from build123d import *

# Parameters (mm, degrees)
BASE_SHAPE_DEPTH                               = 3
EDGE_RADIUSES_R                                = 3.4
CAMERA_MOUNT_HOLES_REACH                       = 5
SKETCH3_R                                      = 1
CSK_FOR_M2_FLAT_HEAD_MACHINE_SCREW1_AT_2_COUNT = 2
CSK_FOR_M2_FLAT_HEAD_MACHINE_SCREW1_AT_2_PITCH = 22
MILLING_RADIUSES_R                             = 1
SKETCH8_R                                      = 0.5
MILLING_CUTS_1MM_DEPTH                         = 3


with BuildPart() as part:
    # Sketch1 → Base shape (new body)
    with BuildSketch(Plane.XY):
        Polygon((15.5, 6), (-15.5, 6), (-15.5, -6), (-14, -6), (-14, -6.9), (-11.05, -6.9), (-11.05, -5.1), (-12.3, -5.1), (-12.3, -2.9), (-7.7, -2.9), (-7.7, -5.1), (-8.95, -5.1), (-8.95, -6.9), (-6, -6.9), (-6, -6), (6, -6), (6, -6.9), (8.95, -6.9), (8.95, -5.1), (7.7, -5.1), (7.7, -2.9), (12.3, -2.9), (12.3, -5.1), (11.05, -5.1), (11.05, -6.9), (14, -6.9), (14, -6), (15.5, -6), align=None)
        with BuildLine():
            Line((-5, -1.5), (-7, -1.5))
            ThreePointArc((-7, -1.5), (-8, -0.5), (-7, 0.5))
            Line((-7, 0.5), (-5, 0.5))
            ThreePointArc((-5, 0.5), (-4, -0.5), (-5, -1.5))
        make_face(mode=Mode.SUBTRACT)
        with BuildLine():
            ThreePointArc((7, 0.5), (8, -0.5), (7, -1.5))
            Line((7, -1.5), (5, -1.5))
            ThreePointArc((5, -1.5), (4, -0.5), (5, 0.5))
            Line((5, 0.5), (7, 0.5))
        make_face(mode=Mode.SUBTRACT)
    extrude(amount=BASE_SHAPE_DEPTH)

    # Edge radiuses
    edge_radiuses_edges = [part.edges().sort_by_distance(p)[0] for p in [
        (-15.5, 6, 1.5),
        (15.5, 6, 1.5),
    ]]
    fillet(edge_radiuses_edges, radius=EDGE_RADIUSES_R)

    # Sketch3 → Camera mount holes (cut, up to next)
    with BuildSketch(Plane(origin=(0, 0, 3), x_dir=(-1, 0, 0), z_dir=(0, 0, -1)), mode=Mode.PRIVATE) as camera_mount_holes_sk1:
        with Locations((-11, 2.25)):
            Circle(SKETCH3_R)
    camera_mount_holes_tool1 = extrude(camera_mount_holes_sk1.sketch, amount=CAMERA_MOUNT_HOLES_REACH, mode=Mode.PRIVATE) & part.part
    add(camera_mount_holes_tool1.solids().sort_by_distance((11, 2.25, 3))[0], mode=Mode.SUBTRACT)
    # Sketch3 → Camera mount holes (cut, up to next)
    with BuildSketch(Plane(origin=(0, 0, 3), x_dir=(-1, 0, 0), z_dir=(0, 0, -1)), mode=Mode.PRIVATE) as camera_mount_holes_sk2:
        with Locations((11, 2.25)):
            Circle(SKETCH3_R)
    camera_mount_holes_tool2 = extrude(camera_mount_holes_sk2.sketch, amount=CAMERA_MOUNT_HOLES_REACH, mode=Mode.PRIVATE) & part.part
    add(camera_mount_holes_tool2.solids().sort_by_distance((-11, 2.25, 3))[0], mode=Mode.SUBTRACT)

    # Sketch5 → CSK for M2 Flat Head Machine Screw1 (revolve, cut)
    with BuildSketch(Plane(origin=(-11, 2.25, 3), x_dir=(0, -1, 0), z_dir=(1, 0, 0))):
        Polygon((0, 0), (0, 3), (1, 3), (1, 1.3), (2, 0.3), (2, 0), align=None)
    csk_for_m2_flat_head_machine_screw1 = revolve(axis=Axis((-11, 2.25, 9.35), (0, 0, -1)), mode=Mode.SUBTRACT)

    # CSK for M2 Flat Head Machine Screw1 at 2: CSK for M2 Flat Head Machine Screw1 ×2
    with Locations(*[(i * CSK_FOR_M2_FLAT_HEAD_MACHINE_SCREW1_AT_2_PITCH, 0, 0) for i in range(1, CSK_FOR_M2_FLAT_HEAD_MACHINE_SCREW1_AT_2_COUNT)]):
        add(csk_for_m2_flat_head_machine_screw1, mode=Mode.SUBTRACT)

    # Milling radiuses
    milling_radiuses_edges = [part.edges().sort_by_distance(p)[0] for p in [
        (-7.7, -5.1, 1.5),
        (-7.7, -2.9, 1.5),
        (-12.3, -2.9, 1.5),
        (-12.3, -5.1, 1.5),
        (12.3, -5.1, 1.5),
        (12.3, -2.9, 1.5),
        (7.7, -2.9, 1.5),
        (7.7, -5.1, 1.5),
    ]]
    fillet(milling_radiuses_edges, radius=MILLING_RADIUSES_R)

    # Sketch8 → Milling cuts 1mm (cut)
    with BuildSketch(Plane(origin=(0, 0, 3), x_dir=(-1, 0, 0), z_dir=(0, 0, -1))):
        with Locations((-14.353553391, -6.353553391)):
            Circle(SKETCH8_R)
        with Locations((14.353553391, -6.353553391)):
            Circle(SKETCH8_R)
        with Locations((-5.646446609, -6.353553391)):
            Circle(SKETCH8_R)
        with Locations((5.646446609, -6.353553391)):
            Circle(SKETCH8_R)
    extrude(amount=MILLING_CUTS_1MM_DEPTH, mode=Mode.SUBTRACT)


solid = part.part
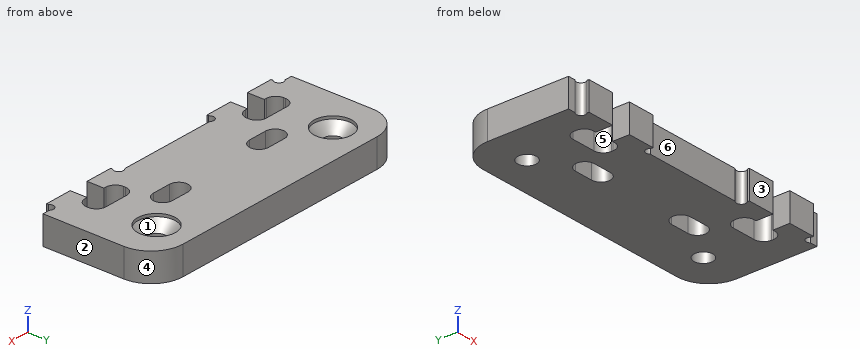
Input: part model. Units: mm. Frame: model coordinates. Face numbers are marked on the shaded views. A direction names the side the tool comes from. Coordinates: 2 decimals unless noted, no trailing zeros. Loops run counter-clockwise (first coordinate to the right, second up) from the corner with the lowest first, then second, coordinate; pieces in that order, holes last. Notation, with made-up numbers: (31, 81) - (72, 81) arc R27 cw to (72, 99) - close; hole circle Ø6 at (67, 47.25). An arc over 180 degrees is marked (long way). Answer in a Markdown table with one row per item. Add a question column.
Item 1: Contact query for flat-ended pins moving along their axis: P1, Ø1.5, axis at x = 0.5, z = 1, coming from the -Y side; P2, Ø0.8, axis at x = -10, z = 1, coming from the -Y side. Output: stop coordinate, or through.
Item 2: Section query A-A on y = -0.5. Return the cut outline in (x, z), then the cut area to 3 significant figures.
Item 3: Line query: line 1 along X through (y, z) = (-5.75, 1.9); line 2 along X through (y, z) = (2.25, 1.2); line 3 along Y through (x, z) = (11, 2.85). Output: solid intervals per line, ascending. Write a range as [from, to].
Item 4: Mould query, pull axis Y, two halves, no side actions, for the marked faces 1, 2 and 3. Classes: released by +Y, released by -Y, zero draft, split by the parting line, or undercut.
Item 5: Section query C-C on x = 2.5. Return the cut outline in (y, z), then the cut area to 3 significant figures.
Item 6: Section query D-D on z = 2.1. State how many separate pieces and enclosed holes the cut face has, then the cut area to 3 significant figures.
Item 7: Access query for the marked faces 4, 5 and 6. Directions: +Z, -Z, +X, -X, +Y, -Y. A direction counts if a zero-diameter tool reaches every point of the face in a straight line with its end or side. Return the directions, or none.
Item 8: Section query B-B on y = 2.25. Return the cut outline in (x, z), then the cut area to 3 significant figures.
Recorded:
| question | item | result |
|---|---|---|
| 1 | P1 | y = -6 |
| 1 | P2 | y = -2.9 |
| 2 | outline | (-15.5, 0) - (-8, 0) - (-8, 3) - (-15.5, 3) - close; (-4, 0) - (4, 0) - (4, 3) - (-4, 3) - close; (8, 0) - (15.5, 0) - (15.5, 3) - (8, 3) - close |
| 2 | area | 69.0 mm^2 |
| 3 | line 1 | [-15.5, -11.05], [-8.95, 8.95], [11.05, 15.5] |
| 3 | line 2 | [-15.5, -12], [-10, 10], [12, 15.5] |
| 3 | line 3 | [-2.9, 0.25], [4.25, 6] |
| 4 | face 1 | undercut |
| 4 | face 2 | zero draft |
| 4 | face 3 | released by -Y |
| 5 | outline | (-6, 0) - (6, 0) - (6, 3) - (-6, 3) - close |
| 5 | area | 36.0 mm^2 |
| 6 | separate pieces | 1 |
| 6 | enclosed holes | 4 |
| 6 | area | 328 mm^2 |
| 7 | face 4 | +Z, -Z, +X, +Y |
| 7 | face 5 | +Z, -Z |
| 7 | face 6 | +Z, -Z, -Y |
| 8 | outline | (-15.5, 0) - (-12, 0) - (-12, 1.7) - (-13, 2.7) - (-13, 3) - (-15.5, 3) - close; (-10, 0) - (10, 0) - (10, 1.7) - (9, 2.7) - (9, 3) - (-9, 3) - (-9, 2.7) - (-10, 1.7) - close; (12, 0) - (15.5, 0) - (15.5, 3) - (13, 3) - (13, 2.7) - (12, 1.7) - close |
| 8 | area | 77.8 mm^2 |
